Read the model definition and answer for the solid it produces. Units are mm, in the model's axes. A direction names the side the tool comes from. Give positions to 0.01 mm unless a question says otherwise; leave off trailing zeros. Order: outer loops, then holes, each group sorted by start corner. A loop starts at its lowest first (then second) coordinate and runs counter-clockwise, first axis right, second up. Notation, with made-up numbers: (5.25, 14) - (40.25, 14) arc R21 cw to (40.25, 31) - close; hole circle Ø9 at (-13.5, -23). An arc over 180 degrees is marked (long way). Write item = value, one per line.
```python
from build123d import *

# Parameters (mm, degrees)
F2_DEPTH = 19.05
F3_R     = 50.8
F4_W     = 88.9
F4_H     = 19.05
F5_DEPTH = 19.05


# Not quite as in the source:
# - a variable given as a bare number and used for a length is read in inches; the dataset says mm whatever the document's units were


with BuildPart() as f2:
    # F1 (on Front) → F2 (new body)
    with BuildSketch(Plane.XZ):
        with BuildLine():
            Line((292.1, 336.55), (158.75, 336.55))
            ThreePointArc((158.75, 336.55), (0, 177.8), (-158.75, 336.55))
            Line((-158.75, 336.55), (-292.1, 336.55))
            Line((-292.1, 336.55), (-292.1, 158.75))
            ThreePointArc((-292.1, 158.75), (-179.8467984866, 112.2532015134), (-133.35, 0))
            ThreePointArc((-133.35, 0), (-179.8467984866, -112.2532015134), (-292.1, -158.75))
            Line((-292.1, -158.75), (-292.1, -336.55))
            Line((-292.1, -336.55), (-158.75, -336.55))
            ThreePointArc((-158.75, -336.55), (0, -177.8), (158.75, -336.55))
            Line((158.75, -336.55), (292.1, -336.55))
            Line((292.1, -336.55), (292.1, -158.75))
            ThreePointArc((292.1, -158.75), (133.35, 0), (292.1, 158.75))
            Line((292.1, 158.75), (292.1, 336.55))
        make_face()
    extrude(amount=F2_DEPTH)

    # F3
    f3_edges = [f2.edges().sort_by_distance(p)[0] for p in [
        (158.75, -9.525, 336.55),
        (-158.75, -9.525, 336.55),
        (292.1, -9.525, 158.75),
        (292.1, -9.525, -158.75),
        (-292.1, -9.525, -158.75),
        (-292.1, -9.525, 158.75),
        (292.1, -9.525, -336.55),
        (-292.1, -9.525, -336.55),
        (292.1, -9.525, 336.55),
        (-292.1, -9.525, 336.55),
    ]]
    fillet(f3_edges, radius=F3_R)

    # F4 (on face) → F5 (join)
    with BuildSketch(Plane(origin=(0, 0, -336.55), x_dir=(1, 0, 0), z_dir=(0, 0, -1))):
        with Locations((-203.2, 9.525)):
            Rectangle(F4_W, F4_H)
        with Locations((203.2, 9.525)):
            Rectangle(F4_W, F4_H)
    extrude(amount=F5_DEPTH)


solid = f2.part
```
1. Section C-C (z = 114.5) is taken. Determine the outline of the cut face in (x, y), and give its area (3 significant figures).
Recorded:
outline = (-182.14, -19.05) - (182.14, -19.05) - (182.14, 0) - (-182.14, 0) - close
area = 6,940 mm^2
2. Section A-A (x = 224) is taken. Determine the outline of the cut face in (y, z).
Recorded:
outline = (-19.05, -355.6) - (0, -355.6) - (0, -143.4) - (-19.05, -143.4) - close; (-19.05, 143.4) - (0, 143.4) - (0, 336.55) - (-19.05, 336.55) - close
3. For faces 1 (the face through (247.65, -9, -346)), 2 (the face through (281.047, -9.658, 171.664)), 3 (the face through (-281.63, -9.66, 172.41)), 4 (the face through (-171.664, -9.658, 325.497)), 5 (the face through (-276.824, -9.658, 322.064)), determine the directions among +Z, -Z, +X, -X, +Y, -Y from which every point of the face is accessible in a straight line to the end or side of a thin tool.
Recorded:
face_1 = -Z, +X, +Y, -Y
face_2 = +X, +Y, -Y
face_3 = -X, +Y, -Y
face_4 = +Z, +Y, -Y
face_5 = +Z, -X, +Y, -Y
4. Straight lines are drawn through the part: L1, parallel to X at y = -13.5, z = 4.5; L2, parallel to X at y = -16.5, z = -298; L3, parallel to X at y = -12.25, z = 195.5. For each, find the intervals that lie inside material, in ascending order. Write a range as [from, to].
Recorded:
L1 = [-133.41, 133.41]
L2 = [-290.6, -154], [154, 290.6]
L3 = [-291.5, -72.85], [72.85, 291.5]
5. Determine the mould class of faces 6 (the face through (292.1, -9, -245)), 7 (the face through (-4, -19.05, -5)), 8 (the face through (158.75, -9, -346)), 9 (the face through (-158.75, -9, -346)) for opening direction X: +X half, -X half, draft (parallel to the pull), parting line (faces both ways), or undercut.
Recorded:
face_6 = +X half
face_7 = draft
face_8 = undercut
face_9 = undercut
6. Section B-B (y = -13.25) is taken. Determine the outline of the cut face in (x, z), and give its area (3 significant figures).
Recorded:
outline = (-292.1, -285.75) arc R50.8 ccw to (-241.3, -336.55) - (-247.65, -336.55) - (-247.65, -355.6) - (-158.75, -355.6) - (-158.75, -336.55) arc R158.75 cw to (158.75, -336.55) - (158.75, -355.6) - (247.65, -355.6) - (247.65, -336.55) - (241.3, -336.55) arc R50.8 ccw to (292.1, -285.75) - (292.1, -203.3) arc R50.8 ccw to (253.62, -154.01) arc R158.75 cw to (253.62, 154.01) arc R50.8 ccw to (292.1, 203.3) - (292.1, 285.75) arc R50.8 ccw to (241.3, 336.55) - (203.3, 336.55) arc R50.8 ccw to (154.01, 298.07) arc R158.75 cw to (-154.01, 298.07) arc R50.8 ccw to (-203.3, 336.55) - (-241.3, 336.55) arc R50.8 ccw to (-292.1, 285.75) - (-292.1, 203.3) arc R50.8 ccw to (-253.62, 154.01) arc R158.75 cw to (-253.62, -154.01) arc R50.8 ccw to (-292.1, -203.3) - close
area = 234,000 mm^2
7. Flat-ended cylindrical pins translate along their axes: pin 1 (2 mm diameter, centred on x = 51.5, y = -9.5, fed in from -Z); pin 2 (2 mm diameter, centred on y = -11.5, z = 197.5, fed in from -X); pin 3 (5 mm diameter, centred on x = 244.5, y = -5, fed in from +Z). Find the tip coordinate at first contact, or state that the pin passes through.
Recorded:
pin_1 = -186.73
pin_2 = -291.87
pin_3 = 336.55
8. Section D-D (x = 75.5) is taken. Determine the outline of the cut face in (y, z).
Recorded:
outline = (-19.05, -196.9) - (0, -196.9) - (0, 196.9) - (-19.05, 196.9) - close
